from build123d import *

# Parameters (mm, degrees)
ESBO_O1_R                = 35
RESSALTO_EXTRUS_O1_DEPTH = 51
RESSALTO_EXTRUS_O2_DEPTH = 45
CHANFRO1_SIZE            = 4
ESBO_O4_R                = 4.25
CORTE_EXTRUS_O1_DEPTH    = 20
ESBO_O5_R                = 3.25
CORTE_EXTRUS_O2_DEPTH    = 36.0000001


with BuildPart() as part:
    # Esboço1 → Ressalto-extrusão1 (new body, symmetric)
    with BuildSketch(Plane.XY):
        Circle(ESBO_O1_R)
    extrude(amount=RESSALTO_EXTRUS_O1_DEPTH, both=True)

    # Esboço3 → Ressalto-extrusão2 (add)
    with BuildSketch(Plane(origin=(0, 0, 0), x_dir=(1, 0, 0), z_dir=(0, 1, 0))):
        with BuildLine():
            Line((-25, -41.5), (25, -41.5))
            ThreePointArc((25, -41.5), (28.535533906, -40.035533906), (30, -36.5))
            Line((30, -36.5), (30, 18.5))
            ThreePointArc((30, 18.5), (28.535533906, 22.035533906), (25, 23.5))
            Line((25, 23.5), (-25, 23.5))
            ThreePointArc((-25, 23.5), (-28.535533906, 22.035533906), (-30, 18.5))
            Line((-30, 18.5), (-30, -36.5))
            ThreePointArc((-30, -36.5), (-28.535533906, -40.035533906), (-25, -41.5))
        make_face()
    extrude(amount=RESSALTO_EXTRUS_O2_DEPTH)

    # Esboço2 → Corte-Revolução1 (revolve, cut)
    with BuildSketch(Plane(origin=(0, 0, 0), x_dir=(0, 0, -1), z_dir=(1, 0, 0)), mode=Mode.PRIVATE) as corte_revolu_o1_sk:
        Polygon((51, 25), (42.2, 25), (42.2, 26.5), (41, 26.5), (41, 25), (16, 25), (16, 20), (-51, 20), (-51, 0), (51, 0), align=None)
    revolve(corte_revolu_o1_sk.sketch.rotate(Axis((0, 0, 52.957916626), (0, 0, -1)), 90), axis=Axis((0, 0, 52.957916626), (0, 0, -1)), mode=Mode.SUBTRACT)  # turned: the seam where the file's is

    # Chanfro1
    chanfro1_edges = [part.edges().sort_by_distance(p)[0] for p in [
        (-35, 0, -51),
    ]]
    chamfer(chanfro1_edges, length=CHANFRO1_SIZE)

    # Esboço4 → Corte-extrusão1 (cut)
    with BuildSketch(Plane(origin=(0, 45, 0), x_dir=(1, 0, 0), z_dir=(0, 1, 0))):
        with Locations(Location((-17.5, 11, 0), (0, 0, 270))):  # turned: the seam where the file's is
            Circle(ESBO_O4_R)
        with Locations(Location((17.5, 11, 0), (0, 0, 90))):  # turned: the seam where the file's is
            Circle(ESBO_O4_R)
        with Locations(Location((17.5, -29, 0), (0, 0, 270))):  # turned: the seam where the file's is
            Circle(ESBO_O4_R)
        with Locations(Location((-17.5, -29, 0), (0, 0, 90))):  # turned: the seam where the file's is
            Circle(ESBO_O4_R)
    extrude(amount=-CORTE_EXTRUS_O1_DEPTH, mode=Mode.SUBTRACT)

    # Esboço5 → Corte-extrusão2 (cut, through all)
    with BuildSketch(Plane(origin=(0, 0, 0), x_dir=(1, 0, 0), z_dir=(0, 1, 0))):
        with Locations(Location((0, -41, 0), (0, 0, 270))):  # turned: the seam where the file's is
            Circle(ESBO_O5_R)
    extrude(amount=-CORTE_EXTRUS_O2_DEPTH, mode=Mode.SUBTRACT)


solid = part.part
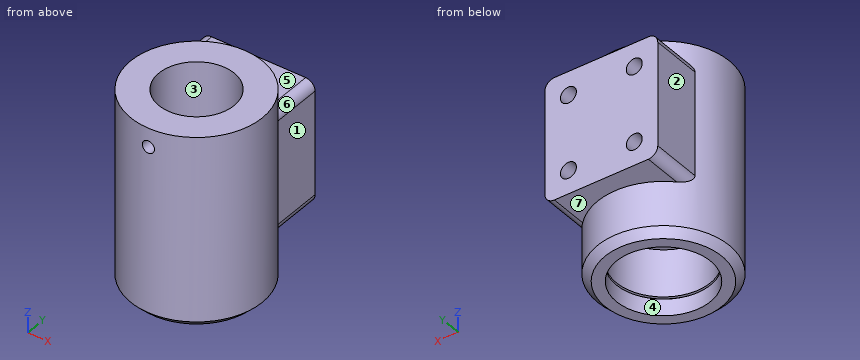
Design review of the part built by this model. Coordinates are the model's own, in mm. Face numbers are marked on the shaded views. A direction names the side the tool comes from. Coordinates: 2 decimals unless noted, no trailing zeros. Order: outer loops, then holes, each group sorted by start corner. A loop starts at its lowest first (then second) coordinate and runs counter-clockwise, first axis right, second up.
Item 1: For the marked faces 4, 5, 6 and 7, list the 3-axis set-ups (+Z, -Z, +X, -X, +Y, -Y) from which the entire face can be reached by the end or side of a thin tool; tool diameter is ignored.
Item 2: The part is to be moulded in two halves that separate along X. For the marked faces 1, 2 and 3, say which applies: pulls with the +X half, pulls with the -X half, needs draft (parallel to the pull), parting line crosses it, or undercut.
Item 3: Take a section at C-C, the plane z = 12. Write out the cut boundary in (x, y).
Item 4: Take a section at B-B, the plane z = 26.5. Write out the cut boundary in (x, y).
Item 5: Take a section at A-A, the plane x = 0. Count the separate pieces of the cut face and the enclosed holes in it, then the cut area to 3 significant figures.
Item 6: Take a section at D-D, the plane z = 43. Write out the cut boundary in (x, y), then the cut area to 3 significant figures.
Item 7: For pin 1 Ø1.5 at (y, z) = (-20, -12) entering from -X; pin 2 Ø1.5 at (x, z) = (-7, 18) entering from -Y; pin 3 Ø7 at (x, z) = (17.5, -11) entering from -Y; pin 4 Ø24 at (x, y) = (0, 0) entering from +Z, all flat-tipped, find the tip position at first contact; note any pin that passes through.
Item 8: For line 1 (X direction, y = 30.25, z = 29); line 2 (Z direction, x = 7, y = 25.5); line 3 (Y direction, x = 0, z = 15), list the stretches that pass through material, from the lowest coordinate up.
The answers:
1. face 4: -Z
1. face 5: +Z, +Y
1. face 6: +Z, +X, +Y
1. face 7: -Z, +Y
2. face 1: pulls with the +X half
2. face 2: pulls with the -X half
2. face 3: undercut
3. outline: (-30, 18.03) arc R35 ccw (long way) to (30, 18.03) - (30, 45) - (-30, 45) - close; hole circle Ø40 at (0, 0)
4. outline: (-30, 18.03) arc R35 ccw (long way) to (30, 18.03) - (30, 45) - (20.94, 45) - (20.94, 25) - (14.06, 25) - (14.06, 45) - (-14.06, 45) - (-14.06, 25) - (-20.94, 25) - (-20.94, 45) - (-30, 45) - close; hole circle Ø40 at (0, 0)
5. separate pieces: 3
5. enclosed holes: 0
5. area: 3,240 mm2
6. outline: (-2.56, -34.91) - (-2.56, -19.84) arc R20 cw (long way) to (2.56, -19.84) - (2.56, -34.91) arc R35 ccw (long way) to start
6. area: 2,510 mm2
7. pin 1: stops at x = -29.23
7. pin 2: stops at y = -34.44
7. pin 3: stops at y = -32.08
7. pin 4: passes through
8. line 1: x = -30 to -21.75, -13.25 to 13.25, 21.75 to 30
8. line 2: z = -51 to -42.2, -41 to 51
8. line 3: y = -35 to -20, 20 to 45
